Drawing for the job (mm, zero at the part's lowest x, y, z). Give positions to 0.01 mm unless a question says otherwise; leave off trailing zeros. Write each loop counter-clockwise with the first axis right and the second up, starting at its lowest first coordinate (ties: lowest second). Pieces come first, ordered by that corner, then holes. Notation, with made-up numbers: M -24.5,-24.5 L 5.5,-24.5 A11 cw 5.5,-19.5 Z; hole C 17,-38 d4. An arc over 180 degrees is marked long. Use CSV: the item, a comma, the result in double quotes. Start each with the question number.
1. Drill centre lines: line 1 along Z through (x, y) = (2.25, 12.7); line 2 along Z through (x, y) = (2.3, 14); line 3 along Z through (x, y) = (0.75, 63.5). Where is each one in solid material? Low to high. Write a range as from..to.
2. Band-saw the part on A-A, the plane z = 101.6. List the corners of the cut face in (x, y) (1 decimal).
3. Drop a flat-ended pin along its axis: pin 1 Ø1 at (x, y) = (2.5, 39) entering from -Z. Give the stop position or say it passes through.
4. Band-saw the part on B-B, the plane z = 63.5. List the corners of the cut face in (x, y) (1 decimal).
5. Band-saw the part on C-C, the plane y = 12.7. List the corners of the cut face in (x, z) (1 decimal).
6. Band-saw the part on D-D, the plane x = 2.45. List the corners of the cut face in (y, z) (1 decimal).
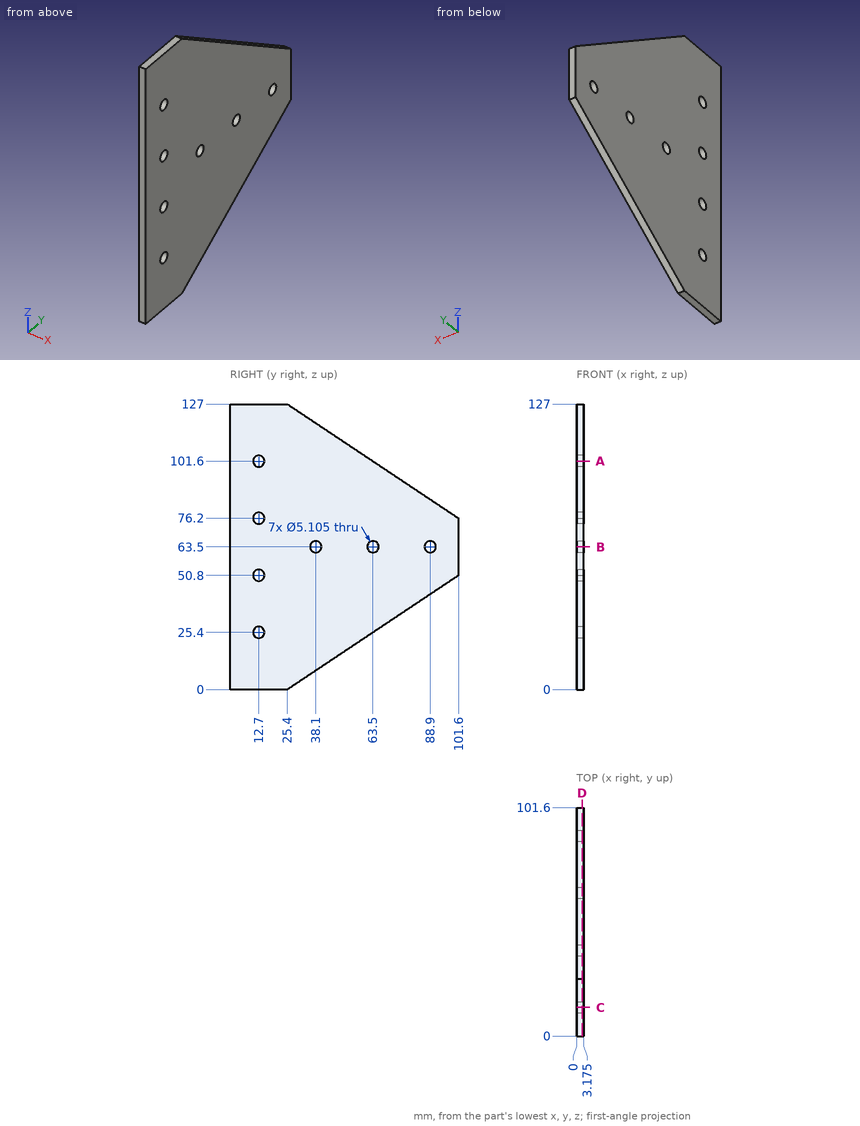
Output:
1,line 1,"z = 0..22.85, 27.95..48.25, 53.35..73.65, 78.75..99.05, 104.15..127"
1,line 2,"z = 0..23.2, 27.6..48.6, 53..74, 78.4..99.4, 103.8..127"
1,line 3,"z = 25.4..60.95, 66.05..101.6"
2,outline,"M 0,0 L 3.2,0 L 3.2,10.1 L 0,10.1 Z; M 0,15.3 L 3.2,15.3 L 3.2,63.5 L 0,63.5 Z"
3,pin 1,"stops at z = 8.73"
4,outline,"M 0,0 L 3.2,0 L 3.2,35.5 L 0,35.5 Z; M 0,40.7 L 3.2,40.7 L 3.2,60.9 L 0,60.9 Z; M 0,66.1 L 3.2,66.1 L 3.2,86.3 L 0,86.3 Z; M 0,91.5 L 3.2,91.5 L 3.2,101.6 L 0,101.6 Z"
5,outline,"M 0,0 L 3.2,0 L 3.2,22.8 L 0,22.8 Z; M 0,28 L 3.2,28 L 3.2,48.2 L 0,48.2 Z; M 0,53.4 L 3.2,53.4 L 3.2,73.6 L 0,73.6 Z; M 0,78.8 L 3.2,78.8 L 3.2,99 L 0,99 Z; M 0,104.2 L 3.2,104.2 L 3.2,127 L 0,127 Z"
6,outline,"M 0,0 L 25.4,0 L 101.6,50.8 L 101.6,76.2 L 25.4,127 L 0,127 Z; hole C 12.7,25.4 d5.1; hole C 12.7,50.8 d5.1; hole C 12.7,76.2 d5.1; hole C 12.7,101.6 d5.1; hole C 38.1,63.5 d5.1; hole C 63.5,63.5 d5.1; hole C 88.9,63.5 d5.1"
